from build123d import *

# Parameters (mm, degrees)
EXTRUDE_DEPTH   = 3.3
SKETCH001_R     = 1.5
POCKET_DEPTH    = 3.301
SKETCH002_R     = 3
POCKET001_DEPTH = 8


with BuildPart() as part:
    # Sketch → Extrude (new body)
    with BuildSketch(Plane.XY):
        with BuildLine():
            ThreePointArc((3.5, 21.5), (0, 25), (-3.5, 21.5))
            Line((-3.5, 21.5), (-3.5, 19.691369))
            ThreePointArc((-3.5, 19.691369), (0, -20), (3.5, 19.691369))
            Line((3.5, 19.691369), (3.5, 21.5))
        make_face()
    extrude(amount=EXTRUDE_DEPTH)

    # Sketch001 (on Face6 of Extrude) → Pocket (cut, through all)
    with BuildSketch(Plane.XY.offset(3.3)):
        with Locations((0, 21.5)):
            Circle(SKETCH001_R)
    extrude(amount=-POCKET_DEPTH, mode=Mode.SUBTRACT)

    # Sketch002 (on Face6 of BaseFeature) → Pocket001 (cut)
    with BuildSketch(Plane.XY.offset(3.3)):
        with Locations((-9, 9)):
            Circle(SKETCH002_R)
        with Locations((9, 9)):
            Circle(SKETCH002_R)
        with BuildLine():
            ThreePointArc((-11.5, -9.63068), (0, -15), (11.5, -9.63068))
            Line((-11.5, -9.63068), (11.5, -9.63068))
        make_face()
    extrude(amount=-POCKET001_DEPTH, mode=Mode.SUBTRACT)


solid = part.part
Geometry check sheet. Reference: the model listing, model coordinates, mm. A direction names the side the tool comes from. Give positions to 0.01 mm unless a question says otherwise; leave off trailing zeros. Loops run counter-clockwise (first coordinate to the right, second up) from the corner with the lowest first, then second, coordinate; pieces in that order, holes last. Notation, with made-up numbers: (15, 36) -> (49, 36) arc R18 ccw to (49, 49) -> close; hole circle Ø8 at (34.25, 22). An arc over 180 degrees is marked (long way). Answer in a Markdown table with one row per item. Add a question column.
1) Cross-section at A-A on x = 0. Record the boundary of the cut face in (y, z).
2) Cross-section at D-D on y = 18. Record the boundary of the cut face in (x, z), and give its area (3 significant figures).
3) Gauge pin test, flat ends, axial feed: P1, Ø1, axis at x = 3.5, z = 1.5, coming from the +Y side; P2, Ø1.5, axis at y = -3, z = 0.5, coming from the -X side; P3, Ø1.4, axis at y = 20.5, z = 1.5, coming from the -X side; P4, Ø2.5, axis at x = 0, y = 21.5, coming from the +Z side. Record the tip position at first contact, or that the pin passes through.
4) Cross-section at C-C on z = 2.3. Record the boundary of the cut face in (x, y), and give its area (3 significant figures).
5) Draft check along Y on faces 4 (the face through (0, -9.631, 2)), 5 (the face through (0, 25, 2)), 6 (the face through (0, 3, 0)). Enter one of: pulls with the +Y half, pulls with the -Y half, needs draft (parallel to the pull), parting line crosses it, or undercut.
6) Cross-section at B-B on y = 9. Record the boundary of the cut face in (x, z), and give its area (3 significant figures).
7) Material ranges on probe 1 along Y at (x, z) = (-7, 0.9) (1 decimal); probe 2 along X at (y, z) = (8.5, 2.75); probe 3 along Y at (x, z) = (8.5, 1.15), recorded low to high. Write a range as from..to.
8) Set-up check for faces 1 (the face through (3.5, 21, 2)), 2 (the face through (0, 3, 3.3)), 3 (the face through (-3.5, 21, 2)): record each of +Z, -Z, +X, -X, +Y, -Y from which the full face is reachable in a straight line by a thin tool's end or side.
Outcome:
| question | item | result |
|---|---|---|
| 1 | outline | (-20, 0) -> (-15, 0) -> (-15, 3.3) -> (-20, 3.3) -> close; (-9.63, 0) -> (20, 0) -> (20, 3.3) -> (-9.63, 3.3) -> close; (23, 0) -> (25, 0) -> (25, 3.3) -> (23, 3.3) -> close |
| 2 | outline | (-8.72, 0) -> (8.72, 0) -> (8.72, 3.3) -> (-8.72, 3.3) -> close |
| 2 | area | 57.5 mm^2 |
| 3 | P1 | stops at y = 23.3 |
| 3 | P2 | stops at x = -19.87 |
| 3 | P3 | stops at x = -3.5 |
| 3 | P4 | passes through |
| 4 | outline | (-3.5, 19.69) arc R20 ccw (long way) to (3.5, 19.69) -> (3.5, 21.5) arc R3.5 ccw to (-3.5, 21.5) -> close; hole circle Ø6 at (-9, 9); hole (-11.5, -9.63) arc R15 ccw to (11.5, -9.63) -> close; hole circle Ø3 at (0, 21.5); hole circle Ø6 at (9, 9) |
| 4 | area | 1,140 mm^2 |
| 5 | face 4 | undercut |
| 5 | face 5 | pulls with the +Y half |
| 5 | face 6 | needs draft |
| 6 | outline | (-17.86, 0) -> (-12, 0) -> (-12, 3.3) -> (-17.86, 3.3) -> close; (-6, 0) -> (6, 0) -> (6, 3.3) -> (-6, 3.3) -> close; (12, 0) -> (17.86, 0) -> (17.86, 3.3) -> (12, 3.3) -> close |
| 6 | area | 78.3 mm^2 |
| 7 | probe 1 | y = -18.7..-13.3, -9.6..6.8, 11.2..18.7 |
| 7 | probe 2 | x = -18.1..-11.96, -6.04..6.04, 11.96..18.1 |
| 7 | probe 3 | y = -18.1..-12.36, -9.63..6.04, 11.96..18.1 |
| 8 | face 1 | +Z, -Z, +X, +Y |
| 8 | face 2 | +Z, +X, -X, +Y, -Y |
| 8 | face 3 | +Z, -Z, -X, +Y |
